```python
from build123d import *

# Parameters (mm, degrees)
SKETCH2_R           = 13.5
BOSS_EXTRUDE1_DEPTH = 32
SKETCH4_R           = 11
CUT_EXTRUDE1_DEPTH  = 10
SKETCH5_R           = 7.5
CUT_EXTRUDE2_DEPTH  = 30
WRAP1_SECTION_W     = 12
WRAP1_SECTION_H     = 2.166
WRAP1_ANGLE         = 109.116628984
CIRPATTERN1_COUNT   = 3


with BuildPart() as part:
    # Sketch2 → Boss-Extrude1 (new body)
    with BuildSketch(Plane.XY):
        Circle(SKETCH2_R)
    extrude(amount=-BOSS_EXTRUDE1_DEPTH)

    # Sketch4 → Cut-Extrude1 (cut)
    with BuildSketch(Plane.XY):
        Circle(SKETCH4_R)
    extrude(amount=-CUT_EXTRUDE1_DEPTH, mode=Mode.SUBTRACT)

    # Sketch5 → Cut-Extrude2 (cut)
    with BuildSketch(Plane.XY):
        Circle(SKETCH5_R)
    extrude(amount=-CUT_EXTRUDE2_DEPTH, mode=Mode.SUBTRACT)

    # Wrap1 section (on wrap section) → Wrap1 (revolve, cut)
    with BuildSketch(Plane(origin=(0, 0, 0), x_dir=(0.9999995414170643, -0.0009576876636740589, 0), z_dir=(-0.0009576876636740589, -0.9999995414170643, 0))):
        with Locations((7.5, -27.667)):
            Rectangle(WRAP1_SECTION_W, WRAP1_SECTION_H)
    wrap1 = revolve(axis=Axis((0, 0, 0), (0, 0, 1)), revolution_arc=WRAP1_ANGLE, mode=Mode.SUBTRACT)

    # CirPattern1: Wrap1 ×3 about axis
    cirpattern1_axis = Axis((0, 0, 0), (0, 0, 1))
    for i in range(1, CIRPATTERN1_COUNT):
        add(wrap1.rotate(cirpattern1_axis, i * 360 / CIRPATTERN1_COUNT), mode=Mode.SUBTRACT)


solid = part.part
```
Read the model definition and answer for the solid it produces. Units are mm, in the model's axes. A direction names the side the tool comes from. Round coordinates to 2 decimals unless told otherwise and drop trailing zeros. Write each loop counter-clockwise with the first axis right and the second up, starting at its lowest first coordinate (ties: lowest second). Pieces come first, ordered by that corner, then holes. Notation, with made-up numbers: (0.5, -0.5) - (6.5, -0.5) arc R29 ccw to (6.5, 35.5) - close; hole circle Ø1 at (40, -18). An arc over 180 degrees is marked (long way). One line per item, written item: value.
Q1. Find section A-A (x = 0). Determine the outline of the cut face in (y, z).
The answers:
outline: (-13.5, -32) - (13.5, -32) - (13.5, -28.75) - (7.5, -28.75) - (7.5, -30) - (-7.5, -30) - (-7.5, -28.75) - (-13.5, -28.75) - close; (-13.5, -26.58) - (-7.5, -26.58) - (-7.5, -10) - (-11, -10) - (-11, 0) - (-13.5, 0) - close; (7.5, -26.58) - (13.5, -26.58) - (13.5, 0) - (11, 0) - (11, -10) - (7.5, -10) - close
Q2. Which of the six approach directions +Z, -Z, +X, -X, +Y, -Y give full straight-line access (tool end or side, diameter ignored) to faces 4 (the flat face through (-10, 0, -28.75)), 5 (the flat face through (-5.238, -9.052, -27.652)), 6 (the cylindrical face through (-2.38, -10.74, -4.93))?
The answers:
face 4: -X
face 5: +X, -Y
face 6: +Z
Q3. For a pull along Y with two mould halves and no side action, classify faces 1 (the flat face through (7.2, 2.6, -10)), 2 (the flat face through (5, -8, -26.584)), 3 (the flat face through (10.268, -1.984, -27.652)) as pulls with the +Y half, pulls with the -Y half, needs draft (parallel to the pull), parting line crosses it, or undercut.
The answers:
face 1: undercut
face 2: needs draft
face 3: pulls with the -Y half
Q4. Straight lines are drawn through the part: line 1 (Y direction, x = 0, z = -15.5); line 2 (Z direction, x = 7.25, y = -2.5); line 3 (Y direction, x = 0, z = -7.5). For each, find the intervals that lie inside material, in ascending order. Write a range as from..to.
The answers:
line 1: y = -13.5..-7.5, 7.5..13.5
line 2: z = -32..-28.75, -26.58..-10
line 3: y = -13.5..-11, 11..13.5
Q5. Find section B-B (z = -27.5). Determine the outline of the cut face in (x, y).
The answers:
outline: (-8.85, -10.2) arc R13.5 ccw to (-6.76, -11.68) - (-3.76, -6.49) arc R7.5 cw to (-4.91, -5.67) - close; (-6.74, 11.7) - (-3.74, 6.5) arc R7.5 cw to (-2.45, 7.09) - (-4.41, 12.76) arc R13.5 ccw to start; (7.36, -1.42) - (13.25, -2.56) arc R13.5 ccw to (13.5, -0.01) - (7.5, -0.01) arc R7.5 cw to start
Q6. Find section D-D (z = -6). Determine the outline of the cut face in (x, y).
The answers:
outline: circle Ø27 at (0, 0); hole circle Ø22 at (0, 0)
Q7. Each of these flat-tipped pins is pushed along its axis until it touches: P1, Ø7, axis at x = 6, y = 4, coming from the +Z side; P2, Ø9, axis at x = 0, y = 0, coming from the +Z side; P3, Ø2, axis at y = 4.5, z = -14.5, coming from the +X side. Where does it stop, or does it pass through?
The answers:
P1: stops at z = -10
P2: stops at z = -30
P3: stops at x = 13.04
Q8. Find section C-C (y = 2). Determine the outline of the cut face in (x, z), and give its area (3 significant figures).
The answers:
outline: (-13.35, -32) - (13.35, -32) - (13.35, -28.75) - (7.23, -28.75) - (7.23, -30) - (-7.23, -30) - (-7.23, -28.75) - (-13.35, -28.75) - close; (-13.35, -26.58) - (-7.23, -26.58) - (-7.23, -10) - (-10.82, -10) - (-10.82, 0) - (-13.35, 0) - close; (7.23, -26.58) - (13.35, -26.58) - (13.35, 0) - (10.82, 0) - (10.82, -10) - (7.23, -10) - close
area: 322 mm2
